from build123d import *

# Parameters (mm, degrees)
SCHIZZO1_R                    = 30
SCHIZZO1_W                    = 10
SCHIZZO1_H                    = 10
ESTRUSIONE_ESTRUSIONE1_DEPTH  = 7.5
TAGLIO_ESTRUSIONE1_DEPTH      = 44.084219849
TAGLIO_ESTRUSIONE1_DEPTH_BACK = 44.084219849


with BuildPart() as part:
    # Schizzo1 → Estrusione-Estrusione1 (new body)
    with BuildSketch(Plane(origin=(0, 0, 0), x_dir=(1, 0, 0), z_dir=(0, 1, 0))):
        with Locations(Location((0, 0, 0), (0, 0, 270))):
            Circle(SCHIZZO1_R)
        Rectangle(SCHIZZO1_W, SCHIZZO1_H, mode=Mode.SUBTRACT)
    extrude(amount=ESTRUSIONE_ESTRUSIONE1_DEPTH)

    # Schizzo2 → Taglio-Estrusione1 (cut, two sides: drawn at the far end of the back side and taken through both)
    with BuildSketch(Plane(origin=(0, 7.5, 0), x_dir=(1, 0, 0), z_dir=(0, 1, 0)).offset(-TAGLIO_ESTRUSIONE1_DEPTH_BACK)):
        with BuildLine():
            Line((-19.887270315, 10.454237391), (-16.532028162, 25.033818024))
            ThreePointArc((-16.532028162, 25.033818024), (-21.93796515, 20.462787813), (-26.122238482, 14.75224243))
            Line((-26.122238482, 14.75224243), (-19.887270315, 10.454237391))
        make_face()
        with BuildLine():
            Line((-22.45, -0.89), (-26.834065376, 13.413908282))
            ThreePointArc((-26.834065376, 13.413908282), (-29.230229034, 6.752311504), (-29.998643344, -0.285302534))
            Line((-29.998643344, -0.285302534), (-22.45, -0.89))
        make_face()
        with BuildLine():
            Line((-18.997270315, -11.995762609), (-29.945936443, -1.800247352))
            ThreePointArc((-29.945936443, -1.800247352), (-28.690276653, -8.76744122), (-25.836935948, -15.246400914))
            Line((-25.836935948, -15.246400914), (-18.997270315, -11.995762609))
        make_face()
        with BuildLine():
            Line((-10.454237391, -19.887270315), (-25.033818024, -16.532028162))
            ThreePointArc((-25.033818024, -16.532028162), (-20.462787813, -21.93796515), (-14.75224243, -26.122238482))
            Line((-14.75224243, -26.122238482), (-10.454237391, -19.887270315))
        make_face()
        with BuildLine():
            ThreePointArc((-13.413908282, -26.834065376), (-6.752311504, -29.230229034), (0.285302534, -29.998643344))
            Line((0.285302534, -29.998643344), (0.89, -22.45))
            Line((0.89, -22.45), (-13.413908282, -26.834065376))
        make_face()
        with BuildLine():
            ThreePointArc((1.800247352, -29.945936443), (8.76744122, -28.690276653), (15.246400914, -25.836935948))
            Line((15.246400914, -25.836935948), (11.995762609, -18.997270315))
            Line((11.995762609, -18.997270315), (1.800247352, -29.945936443))
        make_face()
        with BuildLine():
            ThreePointArc((16.532028162, -25.033818024), (21.93796515, -20.462787813), (26.122238482, -14.75224243))
            Line((26.122238482, -14.75224243), (19.887270315, -10.454237391))
            Line((19.887270315, -10.454237391), (16.532028162, -25.033818024))
        make_face()
        with BuildLine():
            ThreePointArc((30, 0), (29.999660834, 0.14265288), (29.998643344, 0.285302534))
            Line((29.998643344, 0.285302534), (22.45, 0.89))
            Line((22.45, 0.89), (26.834065376, -13.413908282))
            ThreePointArc((26.834065376, -13.413908282), (29.197790681, -6.89122771), (30, 0))
        make_face()
        with BuildLine():
            ThreePointArc((29.945936443, 1.800247352), (28.690276653, 8.76744122), (25.836935948, 15.246400914))
            Line((25.836935948, 15.246400914), (18.997270315, 11.995762609))
            Line((18.997270315, 11.995762609), (29.945936443, 1.800247352))
        make_face()
        with BuildLine():
            Line((14.75224243, 26.122238482), (10.454237391, 19.887270315))
            Line((10.454237391, 19.887270315), (25.033818024, 16.532028162))
            ThreePointArc((25.033818024, 16.532028162), (20.462787813, 21.93796515), (14.75224243, 26.122238482))
        make_face()
        with BuildLine():
            Line((-0.89, 22.45), (13.413908282, 26.834065376))
            ThreePointArc((13.413908282, 26.834065376), (6.752311504, 29.230229034), (-0.285302534, 29.998643344))
            Line((-0.285302534, 29.998643344), (-0.89, 22.45))
        make_face()
        with BuildLine():
            Line((-11.995762609, 18.997270315), (-1.800247352, 29.945936443))
            ThreePointArc((-1.800247352, 29.945936443), (-8.76744122, 28.690276653), (-15.246400914, 25.836935948))
            Line((-15.246400914, 25.836935948), (-11.995762609, 18.997270315))
        make_face()
    extrude(amount=TAGLIO_ESTRUSIONE1_DEPTH + TAGLIO_ESTRUSIONE1_DEPTH_BACK, mode=Mode.SUBTRACT)


solid = part.part
Design review of the part built by this model. Coordinates are the model's own, in mm. A direction names the side the tool comes from. Give positions to 0.01 mm unless a question says otherwise; leave off trailing zeros. Loops run counter-clockwise (first coordinate to the right, second up) from the corner with the lowest first, then second, coordinate; pieces in that order, holes last. Notation, with made-up numbers: M -18.75,-25.5 L 27.25,-25.5 A21 cw 27.25,9.5 Z; hole C -33,21.25 d1. An arc over 180 degrees is marked long. Answer as a JSON object with one key per item and string values.
Item 1: For P1, Ø4, axis at x = -9, y = 5.5, coming from the -Z side, flat-tipped, find the tip position at first contact; note if it passes through.
Output values:
{"P1": "stops at z = -24.36"}
Item 2: Wall thickness on line 1 along Z through (x, y) = (21.5, 1.25); line 2 along Z through (x, y) = (11, 5.75); line 3 along X through (y, z) = (5.25, 22): over which ranges is each line inside the solid? List them lowest first.
Output values:
{"line 1": "z = -17.35 to -13.19, -9.67 to 11.57", "line 2": "z = -26.09 to -20.68, -19.76 to 20.07", "line 3": "x = -11.91 to 9.2, 13.42 to 17.23"}
Item 3: We need section B-B (z = 9). State the section outline as (x, y) points, and give its area (3 significant figures).
Output values:
{"outline": "M -22.21,0 L 25.48,0 L 25.48,7.5 L -22.21,7.5 Z", "area": "358 mm2"}
Item 4: We need section C-C (x = -9). State the section outline as (y, z) points, and give its area (3 significant figures).
Output values:
{"outline": "M 0,-22.21 L 7.5,-22.21 L 7.5,25.48 L 0,25.48 Z", "area": "358 mm2"}
Item 5: Machinability: for faces 1 (the face through (18.233, 3.697, 17.642)), 2 (the face through (-6.969, 3.697, -24.395)), 3 (the face through (-6, 7.5, 0)), 4 (the face through (17.642, 3.697, -18.233)), 5 (the face through (0, 4, 5)), which of the approach directions +Z, -Z, +X, -X, +Y, -Y give a long, thin tool a straight path to every point of the face, cutting with its end or side? Answer none if there is none.
Output values:
{"face 1": "+Z, +Y, -Y", "face 2": "-Z, +Y, -Y", "face 3": "+Z, -Z, +X, -X, +Y", "face 4": "+X, +Y, -Y", "face 5": "+Y, -Y"}
Item 6: Mouldability with a two-part tool opening along Z and no side actions: class faces 6 (the face through (-23, 3.7, -12.6)), 7 (the face through (15.885, 3.698, 25.449)), 8 (the face through (24.61, 3.7, 6.16)) as pulls with the +Z half, pulls with the -Z half, needs draft (parallel to the pull), parting line crosses it, or undercut.
Output values:
{"face 6": "pulls with the -Z half", "face 7": "pulls with the +Z half", "face 8": "undercut"}
Item 7: We need section A-A (x = 2.5). State the section outline as (y, z) points.
Output values:
{"outline": "M 0,-23.49 L 7.5,-23.49 L 7.5,-5 L 0,-5 Z; M 0,5 L 7.5,5 L 7.5,29.19 L 0,29.19 Z"}
